```python
from build123d import *

# Parameters (mm, degrees)
SKETCH1_W            = 28
SKETCH1_H            = 16
BOSS_EXTRUDE1_DEPTH  = 10
SKETCH3_R            = 1.75
CUT_EXTRUDE1_DEPTH   = 10
FILLET5_R            = 3
FILLET6_R            = 3
BOSS_EXTRUDE3_DEPTH  = 10
FILLET7_R            = 0.5
FILLET8_R            = 0.5
SKETCH5_W            = 3.693864044
SKETCH5_H            = 8.2
CUT_EXTRUDE2_DEPTH   = 1
SKETCH7_W            = 0.8
SKETCH7_H            = 7.887258378
BOSS_EXTRUDE5_DEPTH  = 12
SKETCH8_W            = 0.8
SKETCH8_H            = 7.887258378
BOSS_EXTRUDE6_DEPTH  = 12
CHAMFER1_SIZE        = 1
CHAMFER3_SIZE        = 0.2
SKETCH10_R           = 1
CUT_EXTRUDE3_DEPTH   = 8
SKETCH11_W           = 0.8
SKETCH11_H           = 7.887258378
BOSS_EXTRUDE7_DEPTH  = 3
SKETCH12_W           = 0.8
SKETCH12_H           = 7.887258378
BOSS_EXTRUDE8_DEPTH  = 10
FILLET9_R            = 0.5
FILLET10_R           = 0.5
CHAMFER4_SIZE        = 1.5
CHAMFER5_SIZE        = 0.2
SKETCH13_R           = 1
CUT_EXTRUDE4_DEPTH   = 1
SKETCH14_W           = 2.614438376
SKETCH14_H           = 4.181373928
BOSS_EXTRUDE10_DEPTH = 3
FILLET12_R           = 1
SKETCH17_W           = 0.8
SKETCH17_H           = 4.181373928
BOSS_EXTRUDE11_DEPTH = 2.4
BOSS_EXTRUDE12_DEPTH = 4.18
CUT_EXTRUDE9_DEPTH   = 5
FILLET14_R           = 1


with BuildPart() as part:
    # Sketch1 → Boss-Extrude1 (new body)
    with BuildSketch(Plane(origin=(0, 0, 0), x_dir=(1, 0, 0), z_dir=(0, 1, 0))):
        with Locations((14, 8)):
            Rectangle(SKETCH1_W, SKETCH1_H)
    extrude(amount=BOSS_EXTRUDE1_DEPTH)

    # Sketch3 → Cut-Extrude1 (cut)
    with BuildSketch(Plane(origin=(0, 10, 0), x_dir=(1, 0, 0), z_dir=(0, 1, 0))):
        with Locations(Location((2.9, 13.1, 0), (0, 0, 270))):
            Circle(SKETCH3_R)
        with Locations(Location((25.1, 2.9, 0), (0, 0, 270))):
            Circle(SKETCH3_R)
    extrude(amount=-CUT_EXTRUDE1_DEPTH, mode=Mode.SUBTRACT)

    # Fillet5
    fillet5_edges = [part.edges().sort_by_distance(p)[0] for p in [
        (0, 5, -16),
        (28, 5, 0),
    ]]
    fillet(fillet5_edges, radius=FILLET5_R)

    # Fillet6
    fillet6_edges = [part.edges().sort_by_distance(p)[0] for p in [
        (28, 5, -16),
        (0, 5, 0),
    ]]
    fillet(fillet6_edges, radius=FILLET6_R)

    # Sketch4 → Boss-Extrude3 (add)
    with BuildSketch(Plane(origin=(0, 10, 0), x_dir=(1, 0, 0), z_dir=(0, 1, 0))):
        Polygon((0, 10.651040916), (-1.949468991, 9.930649363), (-1.949468991, 6.357507258), (-0.974734495, 6.357507258), (-0.974734495, 4.369226571), (0.098482911, 3.762363811), align=None)
    extrude(amount=-BOSS_EXTRUDE3_DEPTH)

    # Fillet7
    fillet7_edges = [part.edges().sort_by_distance(p)[0] for p in [
        (-1.949468991, 5, -9.930649363),
    ]]
    fillet(fillet7_edges, radius=FILLET7_R)

    # Fillet8
    fillet8_edges = [part.edges().sort_by_distance(p)[0] for p in [
        (-1.949468991, 5, -6.357507258),
    ]]
    fillet(fillet8_edges, radius=FILLET8_R)

    # Sketch5 → Cut-Extrude2 (cut)
    with BuildSketch(Plane.ZY.offset(1.949468991)):
        with Locations((-8.20443928, 5)):
            Rectangle(SKETCH5_W, SKETCH5_H)
    extrude(amount=-CUT_EXTRUDE2_DEPTH, mode=Mode.SUBTRACT)

    # Sketch7 → Boss-Extrude5 (add)
    with BuildSketch(Plane.ZY.offset(0.949468991)):
        with Locations((-9.651371302, 5.008233046)):
            Rectangle(SKETCH7_W, SKETCH7_H)
    extrude(amount=BOSS_EXTRUDE5_DEPTH)

    # Sketch8 → Boss-Extrude6 (add)
    with BuildSketch(Plane.ZY.offset(0.974734495)):
        with Locations((-4.769226571, 5.008233046)):
            Rectangle(SKETCH8_W, SKETCH8_H)
    extrude(amount=BOSS_EXTRUDE6_DEPTH)

    # Chamfer1
    chamfer1_edges = [part.edges().sort_by_distance(p)[0] for p in [
        (-12.949468991, 1.064603857, -9.651371302),
        (-12.949468991, 8.951862235, -9.651371302),
        (-12.974734495, 8.951862235, -4.769226571),
        (-12.974734495, 1.064603857, -4.769226571),
    ]]
    chamfer(chamfer1_edges, length=CHAMFER1_SIZE)

    # Chamfer3
    chamfer3_edges = [part.edges().sort_by_distance(p)[0] for p in [
        (-12.949468991, 5.008233046, -10.051371302),
        (-12.949468991, 5.008233046, -9.251371302),
        (-12.449468991, 8.451862235, -9.251371302),
        (-12.449468991, 1.564603857, -9.251371302),
        (-12.449468991, 8.451862235, -10.051371302),
        (-12.449468991, 1.564603857, -10.051371302),
        (-12.974734495, 5.008233046, -4.369226571),
        (-12.974734495, 5.008233046, -5.169226571),
        (-12.474734495, 8.451862235, -4.369226571),
        (-12.474734495, 1.564603857, -4.369226571),
        (-12.474734495, 8.451862235, -5.169226571),
        (-12.474734495, 1.564603857, -5.169226571),
    ]]
    chamfer(chamfer3_edges, length=CHAMFER3_SIZE)

    # Sketch10 → Cut-Extrude3 (cut)
    with BuildSketch(Plane.XY.offset(-4.369226571)):
        with Locations((-7.774734495, 5.008233046)):
            Circle(SKETCH10_R)
    extrude(amount=-CUT_EXTRUDE3_DEPTH, mode=Mode.SUBTRACT)

    # Sketch11 → Boss-Extrude7 (add)
    with BuildSketch(Plane.XY):
        with Locations((11.855374497, 5.008233046)):
            Rectangle(SKETCH11_W, SKETCH11_H)
    extrude(amount=BOSS_EXTRUDE7_DEPTH)

    # Sketch12 → Boss-Extrude8 (add)
    with BuildSketch(Plane.ZY.offset(-11.455374497)):
        with Locations((2.6, 5.008233046)):
            Rectangle(SKETCH12_W, SKETCH12_H)
    extrude(amount=BOSS_EXTRUDE8_DEPTH)

    # Fillet9
    fillet9_edges = [part.edges().sort_by_distance(p)[0] for p in [
        (11.455374497, 5.008233046, 2.2),
    ]]
    fillet(fillet9_edges, radius=FILLET9_R)

    # Fillet10
    fillet10_edges = [part.edges().sort_by_distance(p)[0] for p in [
        (12.255374497, 5.008233046, 3),
    ]]
    fillet(fillet10_edges, radius=FILLET10_R)

    # Chamfer4
    chamfer4_edges = [part.edges().sort_by_distance(p)[0] for p in [
        (1.455374497, 8.951862235, 2.6),
        (1.455374497, 1.064603857, 2.6),
    ]]
    chamfer(chamfer4_edges, length=CHAMFER4_SIZE)

    # Chamfer5
    chamfer5_edges = [part.edges().sort_by_distance(p)[0] for p in [
        (1.455374497, 5.008233046, 3),
        (1.455374497, 5.008233046, 2.2),
        (2.205374497, 8.201862235, 3),
        (2.205374497, 1.814603857, 3),
        (2.205374497, 8.201862235, 2.2),
        (2.205374497, 1.814603857, 2.2),
    ]]
    chamfer(chamfer5_edges, length=CHAMFER5_SIZE)

    # Sketch13 → Cut-Extrude4 (cut)
    with BuildSketch(Plane.XY.offset(3)):
        with Locations((6.455374497, 5.008233046)):
            Circle(SKETCH13_R)
    extrude(amount=-CUT_EXTRUDE4_DEPTH, mode=Mode.SUBTRACT)

    # Sketch14 → Boss-Extrude10 (add)
    with BuildSketch(Plane(origin=(0, 0, -16), x_dir=(-1, 0, 0), z_dir=(0, 0, -1))):
        with Locations((-22.392780812, 5)):
            Rectangle(SKETCH14_W, SKETCH14_H)
    extrude(amount=BOSS_EXTRUDE10_DEPTH)

    # Fillet12
    fillet12_edges = [part.edges().sort_by_distance(p)[0] for p in [
        (23.7, 5, -19),
        (21.085561624, 5, -19),
    ]]
    fillet(fillet12_edges, radius=FILLET12_R)

    # Sketch17 → Boss-Extrude11 (add)
    with BuildSketch(Plane(origin=(0, 0, -16), x_dir=(-1, 0, 0), z_dir=(0, 0, -1))):
        with Locations((-11.087924536, 5)):
            Rectangle(SKETCH17_W, SKETCH17_H)
    extrude(amount=BOSS_EXTRUDE11_DEPTH)

    # Sketch18 → Boss-Extrude12 (add)
    with BuildSketch(Plane(origin=(0, 7.090686964, 0), x_dir=(1, 0, 0), z_dir=(0, 1, 0))):
        Polygon((60.18861552, 25.33460318), (11.487924536, 18.4), (11.487924536, 17.599656508), (60.18861552, 24.534259688), align=None)
    extrude(amount=-BOSS_EXTRUDE12_DEPTH)

    # Sketch20 → Cut-Extrude9 (cut)
    with BuildSketch(Plane(origin=(0, 7.090686964, 0), x_dir=(1, 0, 0), z_dir=(0, 1, 0))):
        Polygon((11.956915688, 18.464207931), (10.687924536, 18.283513368), (10.687924536, 18.4), align=None)
    extrude(amount=-CUT_EXTRUDE9_DEPTH, mode=Mode.SUBTRACT)

    # Fillet14
    fillet14_edges = [part.edges().sort_by_distance(p)[0] for p in [
        (11.487924536, 5.000686964, -17.599656508),
    ]]
    fillet(fillet14_edges, radius=FILLET14_R)


solid = part.part
```
Could you check a few things on this model? Use its own coordinates, in mm. A direction names the side the tool comes from. Give positions to 0.01 mm unless a question says otherwise; leave off trailing zeros. Order: outer loops, then holes, each group sorted by start corner. A loop starts at its lowest first (then second) coordinate and runs counter-clockwise, first axis right, second up.
Q1. I'm going to push flat-ended pins straight in: P1, Ø2, axis at x = 0.5, y = 8, coming from the -Z side; P2, Ø0.6, axis at x = -7.5, z = -10, coming from the +Y side; P3, Ø3, axis at x = 13.5, y = 6, coming from the -Z side; P4, Ø3.5, axis at x = 6, z = 1, coming from the +Y side. Where does each tip first touch, or does it pass through?
Q2. We'd pull the mould along Y, two halves only. Please class faces 1 (the flat face through (14, 5, 0)), 2 (the flat face through (-0.949, 5, -8)), 3 (the flat face through (35.3, 7.091, -21.4)), 4 (the cylindrical face through (-6.85, 4.63, -4.76)): +Y half, -Y half, draft (parallel to the pull), parting line (faces both ways), or undercut.
Q3. If I drill on line 1 along X through (y, z) = (3, -13.1); line 2 along X through (y, z) = (2.5, -2.9); line 3 along Y through (x, z) = (-2, -4.5), over which ranges is the centre line in solid material (lowest first)?
Q4. For faces 5 (the flat face through (2.216, 8.212, 2.597)), 6 (the flat face through (8.7, 1.065, 2.5)), which set-ups out of +Z, -Z, +X, -X, +Y, -Y let a thin tool reach every point of the face, with its end or its side?
Q5. Suppose I cut it at A-A, the plane x = 10. Write out the boundary of the cut face in (y, z), and give its area (3 significant figures).
Solution:
1. P1: stops at z = -15.6
1. P2: stops at y = 8.95
1. P3: stops at z = -18.9
1. P4: stops at y = 10
2. face 1: draft
2. face 2: undercut
2. face 3: +Y half
2. face 4: undercut
3. line 1: x = 0 to 1.15, 4.65 to 28
3. line 2: x = 0 to 23.35, 26.85 to 28
3. line 3: y = 1.06 to 8.95
4. face 5: +Z, -X, +Y
4. face 6: +Z, +X, -X, -Y
5. outline: (0, -16) - (10, -16) - (10, 0) - (0, 0) - close; (1.06, 2.2) - (8.95, 2.2) - (8.95, 3) - (1.06, 3) - close
5. area: 166 mm2
